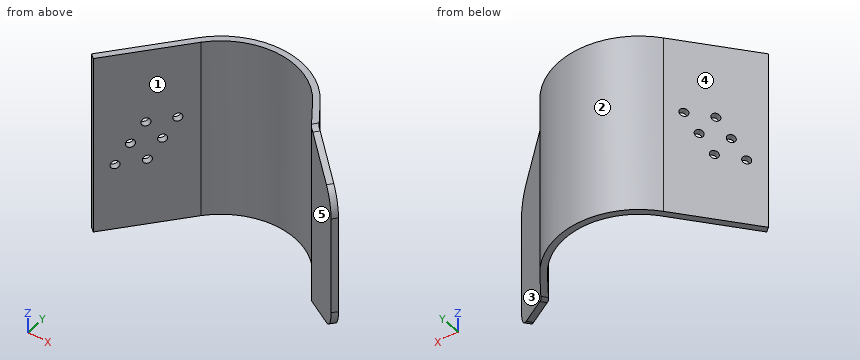
```python
from build123d import *

# Parameters (mm, degrees)
ESTRUSIONE_SOTTILE1_START = -37
ESTRUSIONE_SOTTILE1_DEPTH = 74
SCHIZZO2_R                = 1.7
TAGLIO_ESTRUSIONE2_DEPTH  = 23
TAGLIO_ESTRUSIONE4_DEPTH  = 10
RACCORDO1_R               = 10


# Read off the part's stored shape, not the designer's step: Estrusione-Sottile1
with BuildPart() as part:
    # Estrusione-Sottile1 outline → Estrusione-Sottile1 (new body)
    with BuildSketch(Plane.XY.offset(ESTRUSIONE_SOTTILE1_START)):
        with BuildLine():
            ThreePointArc((75.309556173, 93.111427552), (99.681203079, 103.663061306), (122.974907994, 90.906985924))
            Line((122.974907994, 90.906985924), (130.786083182, 79.848715119))
            Line((130.786083182, 79.848715119), (152.209243946, 62.072969532))
            Line((152.209243946, 62.072969532), (153.805626203, 63.996914357))
            Line((153.805626203, 63.996914357), (132.637123428, 81.561358928))
            Line((132.637123428, 81.561358928), (125.016863249, 92.349351598))
            ThreePointArc((125.016863249, 92.349351598), (99.3221362, 106.178890254), (72.802722922, 94.005318182))
            Line((72.802722922, 94.005318182), (50.135913498, 66.687493457))
            Line((50.135913498, 66.687493457), (52.059858323, 65.0911112))
            Line((52.059858323, 65.0911112), (75.309556173, 93.111427552))
        make_face()
    extrude(amount=ESTRUSIONE_SOTTILE1_DEPTH)

    # Schizzo2 → Taglio-Estrusione2 (cut)
    with BuildSketch(Plane(origin=(-1.154366895, 0.957829354, 0), x_dir=(0, 0, -1), z_dir=(0.76957792998473, -0.6385529028047858, 0))):
        with Locations(Location((-6.552412565, 111.975385882, 0), (0, 0, 90))):
            Circle(SCHIZZO2_R)
        with Locations(Location((-6.552412565, 101.158520834, 0), (0, 0, 90))):
            Circle(SCHIZZO2_R)
        with Locations(Location((1.452296176, 106.816436865, 0), (0, 0, 90))):
            Circle(SCHIZZO2_R)
        with Locations(Location((9.457004918, 101.657487848, 0), (0, 0, 90))):
            Circle(SCHIZZO2_R)
        with Locations(Location((1.553386665, 95.93442008, 0), (0, 0, 90))):
            Circle(SCHIZZO2_R)
        with Locations(Location((9.659185895, 90.710319326, 0), (0, 0, 90))):
            Circle(SCHIZZO2_R)
    extrude(amount=-TAGLIO_ESTRUSIONE2_DEPTH, mode=Mode.SUBTRACT)

    # Schizzo3 → Taglio-Estrusione4 (cut)
    with BuildSketch(Plane(origin=(94.163336629, 113.484764324, 0), x_dir=(0.769577929984725, -0.6385529028047917, 0), z_dir=(0.6385529028047917, 0.769577929984725, 0))):
        Polygon((49.993360387, -37), (77.5, -27), (77.5, -37), align=None)
        Polygon((49.993360387, 37), (77.5, 27), (77.5, 37), align=None)
    extrude(amount=-TAGLIO_ESTRUSIONE4_DEPTH, mode=Mode.SUBTRACT)

    # Raccordo1
    raccordo1_edges = [part.edges().sort_by_distance(p)[0] for p in [
        (131.8389323, 80.599386516, -37),
        (131.8389323, 80.599386516, 37),
        (153.007435074, 63.034941944, -27),
        (153.007435074, 63.034941944, 27),
    ]]
    fillet(raccordo1_edges, radius=RACCORDO1_R)


solid = part.part
```
Source: CAD feature listing. Evaluate the final solid. Frame: model axes, mm. Face numbers are marked on the shaded views. A direction names the side the tool comes from. Give positions to 0.01 mm unless a question says otherwise; leave off trailing zeros. Write each loop counter-clockwise with the first axis right and the second up, starting at its lowest first coordinate (ties: lowest second). Pieces come first, ordered by that corner, then holes.
1. Section query C-C (x = 95). Return the cut outline in (y, z), then the cut area to 3 significant figures.
2. Access query for the marked faces 4 and 5. Directions: +Z, -Z, +X, -X, +Y, -Y. A direction counts if a zero-diameter tool reaches every point of the face in a straight line with its end or side. Return the directions, or none.
3. Section query D-D (x = 145). Return the cut outline in (y, z), then the cut area to 3 significant figures.
4. First-contact query: pin 1 (8 mm diameter, centred on x = 78.5, z = 4, fed in from +Y); pin 2 (1.5 mm diameter, centred on x = 99, z = -24, fed in from +Y); pin 3 (1.5 mm diameter, centred on x = 140.5, z = -21, fed in from -Y); pin 4 (3 mm diameter, centred on y = 67.5, z = 19.5, fed in from -X). Flat tips, straight axial feed; report the tip coordinate or a pass-through.
5. Section query B-B (z = -23). Return the cut outline in (x, y), then the cut area to 3 significant figures.
6. Section query A-A (y = 100.5). Return the cut outline in (x, z), then the cut area to 4 significant figures.
7. Material intervals for line 1 along X through (y, z) = (83, 30.5); line 2 along X through (y, z) = (78, 15); line 3 along Y through (x, z) = (142.5, 17), sorted ascending.
8. Pull-direction query (X, two-part tool) for the marked faces 1, 2 and 3; classes: +X half, -X half, draft (parallel to the pull), parting line (faces both ways), or undercut.
Output values:
1. outline: (103.52, -37) - (106.03, -37) - (106.03, 37) - (103.52, 37) - close
1. area: 186 mm2
2. face 4: +Z, -Z, -X, +Y
2. face 5: +Z, -Z, -Y
3. outline: (68.05, -30.41) - (71.3, -31.16) - (71.3, 31.16) - (68.05, 30.41) - close
3. area: 200 mm2
4. pin 1: stops at y = 102.14
4. pin 2: stops at y = 106.2
4. pin 3: stops at y = 71.17
4. pin 4: stops at x = 50.14
5. outline: (50.14, 66.69) - (52.06, 65.09) - (75.31, 93.11) arc R30.23 cw to (122.97, 90.91) - (130.79, 79.85) - (151.85, 62.37) - (153.45, 64.29) - (132.64, 81.56) - (125.02, 92.35) arc R32.73 ccw to (72.8, 94.01) - close
5. area: 336 mm2
6. outline: (79.84, -37) - (84.76, -37) - (84.76, 37) - (79.84, 37) - close; (111.81, -37) - (116.73, -37) - (116.73, 37) - (111.81, 37) - close
6. area: 728.5 mm2
7. line 1: x = 63.67 to 66.92, 128.56 to 131.62
7. line 2: x = 59.52 to 62.77, 133.01 to 136.93
7. line 3: y = 70.13 to 73.38
8. face 1: undercut
8. face 2: parting line
8. face 3: +X half
